```python
from build123d import *


with BuildPart() as part:
    # Sketch1 → Revolve1 (revolve)
    with BuildSketch(Plane.XY, mode=Mode.PRIVATE) as revolve1_sk:
        with BuildLine():
            Line((-2.5, 0), (-7.5, 0))
            Line((-7.5, 0), (-7.5, 0.5))
            ThreePointArc((-7.5, 0.5), (-6.158312395, 3), (-7.5, 5.5))
            Line((-7.5, 5.5), (-7.5, 6))
            Line((-7.5, 6), (-3.65, 6))
            Line((-3.65, 6), (-3.65, 1))
            Line((-3.65, 1), (-2.5, 1))
            Line((-2.5, 1), (-2.5, 0))
        make_face()
    revolve(revolve1_sk.sketch.rotate(Axis((0, -6.629530881, 0), (0, 1, 0)), 270), axis=Axis((0, -6.629530881, 0), (0, 1, 0)))


solid = part.part
```
Verification items for the finished model (mm, model axes). A direction names the side the tool comes from. Give positions to 0.01 mm unless a question says otherwise; leave off trailing zeros. Loops run counter-clockwise (first coordinate to the right, second up) from the corner with the lowest first, then second, coordinate; pieces in that order, holes last.
1. Section check D-D, the plane y = 3. Enter the section's corners in (x, z).
2. Thickness scan on line 1 (X direction, y = 0.4, z = 0); line 2 (Y direction, x = 2.5, z = 2.5); line 3 (Y direction, x = 5.5, z = 4.25). Record the ranges inside material, lowest first.
3. Mould release check, pull along X, two halves, no side actions. Record for faces 3 (the flat face through (2, 1, -2)), 4 (the cylindrical face through (-0.33, 0.254, 7.493)), 5 (the flat face through (-2, 0, -2)): released by +X, released by -X, zero draft, split by the parting line, or undercut.
4. Section check A-A, the plane z = 0. Enter the section's corners in (x, y), then the cut area to 3 significant figures.
5. Set-up check for faces 1 (the cylindrical face through (-0.33, 5.754, 7.493)), 2 (the cylindrical face through (1.4, 3.47, -3.37)): record each of +Z, -Z, +X, -X, +Y, -Y from which the full face is reachable in a straight line by a thin tool's end or side.
6. Section check C-C, the plane y = 4. Enter the section's corners in (x, z), then the cut area to 3 significant figures.
7. Go/stop test with flat-tipped pins: pin 1 Ø4 at (x, z) = (0, 0) entering from +Y; pin 2 Ø3 at (x, y) = (5, 5.5) entering from -Z; pin 3 Ø3 at (y, z) = (4.5, -3) entering from -X; pin 4 Ø3 at (x, y) = (-4.5, 3.5) entering from +Z. Record where each tip stops, or that it passes through.
8. Section check B-B, the plane x = 0. Enter the section's corners in (y, z).
Geometry says:
1. outline: circle Ø12.32 at (0, 0); hole circle Ø7.3 at (0, 0)
2. line 1: x = -7.5 to -2.5, 2.5 to 7.5
2. line 2: y = 0 to 1
2. line 3: y = 0 to 0.97, 5.03 to 6
3. face 3: undercut
3. face 4: split by the parting line
3. face 5: zero draft
4. outline: (-7.5, 0) - (-2.5, 0) - (-2.5, 1) - (-3.65, 1) - (-3.65, 6) - (-7.5, 6) - (-7.5, 5.5) arc R3 cw to (-7.5, 0.5) - close; (2.5, 0) - (7.5, 0) - (7.5, 0.5) arc R3 cw to (7.5, 5.5) - (7.5, 6) - (3.65, 6) - (3.65, 1) - (2.5, 1) - close
4. area: 39.1 mm2
5. face 1: +Y, -Y
5. face 2: +Y
6. outline: circle Ø12.66 at (0, 0); hole circle Ø7.3 at (0, 0)
6. area: 84.0 mm2
7. pin 1: passes through
7. pin 2: stops at z = -6.63
7. pin 3: stops at x = -7.26
7. pin 4: stops at z = 5.64
8. outline: (0, -7.5) - (0.5, -7.5) arc R3 cw to (5.5, -7.5) - (6, -7.5) - (6, -3.65) - (1, -3.65) - (1, -2.5) - (0, -2.5) - close; (0, 2.5) - (1, 2.5) - (1, 3.65) - (6, 3.65) - (6, 7.5) - (5.5, 7.5) arc R3 cw to (0.5, 7.5) - (0, 7.5) - close
